Design review of the part built by this model. Coordinates are the model's own, in mm. A direction names the side the tool comes from. Round coordinates to 2 decimals unless told otherwise and drop trailing zeros. Loops run counter-clockwise (first coordinate to the right, second up) from the corner with the lowest first, then second, coordinate; pieces in that order, holes last. Notation, with made-up numbers: M 10,-29.75 L 41,-29.75 A37 ccw 41,9.25 Z; hole C 9,61 d8. An arc over 180 degrees is marked long. One line per item, written item: value. Start each with the question number.
Item 1: We need section A-A (x = 0). Write out the cut boundary in (y, z), then the cut area to 3 significant figures.
Item 2: Clearance check with flat-ended pins moving along their axes: pin 1 (3 mm diameter, centred on y = -6, z = 4.5, fed in from +X); pin 2 (2 mm diameter, centred on y = -6.5, z = 5, fed in from -X); pin 3 (6 mm diameter, centred on x = 8, z = 2.5, fed in from +Y). State where each tip first meets the part, or that it passes through.
Item 3: For faces 1 (the flat face through (3.4, -1.7, 10)), 2 (the cylindrical face through (-2.17, -9.76, 3.94)), list the 3-axis set-ups (+Z, -Z, +X, -X, +Y, -Y) from which the entire face can be reached by the end or side of a thin tool; tool diameter is ignored.
Item 4: For line 1 along Y through (x, z) = (0, 3.75); line 2 along X through (y, z) = (0, -2.1), list the stretches that pass through material, from the lowest coordinate up.
Item 5: Mouldability with a two-part tool opening along Z and no side actions: class faces 3 (the cylindrical face through (-1.08, 4.88, -2.49)), 4 (the flat face through (-0.1, 5.2, -2)), 5 (the flat face through (-5, -9, 0)) as released by +Z, released by -Z, zero draft, split by the parting line, or undercut.
Item 6: We need section D-D (z = -0.5). Write out the cut boundary in (x, y), then the cut area to 3 significant figures.
Item 7: We need section C-C (z = 3.75). Write out the cut boundary in (x, y), then the cut area to 3 significant figures.
from build123d import *

# Parameters (mm, degrees)
F0_R      = 10
F1_DEPTH  = 8
F2_R      = 12
F2_R_2    = 10
F3_DEPTH  = 2
F4_R      = 12
F4_R_2    = 10
F5_DEPTH  = 2
F6_R      = 3
F7_DEPTH  = 25
F9_R      = 5
F9_R_2    = 3
F10_DEPTH = 1
F11_R     = 0.5
F13_R     = 0.5


# Not quite as in the source:
# - a fillet or chamfer that OpenCascade refuses, or shapes differently, is made with other operations: its cross-section is extruded or revolved along the edge and cut away or added


with BuildPart() as f1:
    # F0 (on Top) → F1 (new body)
    with BuildSketch(Plane.XY):
        Circle(F0_R)
    extrude(amount=F1_DEPTH)

    # F2 (on face) → F3 (join)
    with BuildSketch(Plane.XY.offset(8)):
        Circle(F2_R)
        Circle(F2_R_2, mode=Mode.SUBTRACT)
        Circle(F2_R_2)
    extrude(amount=F3_DEPTH)

    # F4 (on face) → F5 (join)
    with BuildSketch(Plane(origin=(0, 0, 0), x_dir=(1, 0, 0), z_dir=(0, 0, -1))):
        Circle(F4_R)
        Circle(F4_R_2, mode=Mode.SUBTRACT)
        Circle(F4_R_2)
    extrude(amount=F5_DEPTH)

    # F6 (on face) → F7 (cut)
    with BuildSketch(Plane(origin=(0, 0, -2), x_dir=(1, 0, 0), z_dir=(0, 0, -1))):
        Circle(F6_R)
    extrude(amount=-F7_DEPTH, mode=Mode.SUBTRACT)

    # F8: union 

    # F9 (on face) → F10 (join)
    with BuildSketch(Plane(origin=(0, 0, -2), x_dir=(1, 0, 0), z_dir=(0, 0, -1))):
        Circle(F9_R)
        Circle(F9_R_2, mode=Mode.SUBTRACT)
    extrude(amount=F10_DEPTH)

    # F11
    f11_edges = [f1.edges().sort_by_distance(p)[0] for p in [
        (-3, 0, -3),
    ]]
    fillet(f11_edges, radius=F11_R)

    # F12: fillet of radius 5 on 2 edges, made by hand

    # F12_s1 → F12_t2 (revolve, cut)
    with BuildSketch(Plane.XZ):
        with BuildLine():
            ThreePointArc((8, -2), (10.2360679775, -1.472135955), (12, 0))
            Line((12, 0), (12, -2))
            Line((12, -2), (8, -2))
        make_face()
    revolve(axis=Axis((0, 0, -2), (0, 0, -1)), mode=Mode.SUBTRACT)

    # F12_s3 → F12_t4 (revolve, cut)
    with BuildSketch(Plane.XZ):
        with BuildLine():
            ThreePointArc((8, 10), (10.2360679775, 9.472135955), (12, 8))
            Line((12, 8), (12, 10))
            Line((12, 10), (8, 10))
        make_face()
    revolve(axis=Axis((0, 0, 10), (0, 0, 1)), mode=Mode.SUBTRACT)

    # F13
    f13_edges = [f1.edges().sort_by_distance(p)[0] for p in [
        (3, 0, 4),
        (-3, 0, 10),
        (-3, 0, -2),
        (3, 0, -2.25),
        (-3, 0, -2.5),
    ]]
    fillet(f13_edges, radius=F13_R)


solid = f1.part
A:
1. outline: M -12,0 A5 ccw -8,-2 L -5,-2 L -5,-3 L -3.5,-3 A0.5 ccw -3,-2.5 L -3,9.5 A0.5 ccw -3.5,10 L -8,10 A5 ccw -12,8 L -10,8 L -10,0 Z; M 3,-2.5 A0.5 ccw 3.5,-3 L 5,-3 L 5,-2 L 8,-2 A5 ccw 12,0 L 10,0 L 10,8 L 12,8 A5 ccw 8,10 L 3.5,10 A0.5 ccw 3,9.5 Z
1. area: 178 mm2
2. pin 1: x = 8.93
2. pin 2: x = -8.35
2. pin 3: y = 10.19
3. face 1: +Z, +X, -X, +Y, -Y
3. face 2: none
4. line 1: -10 to -3, 3 to 10
4. line 2: -5 to -3, 3 to 5
5. face 3: zero draft
5. face 4: released by -Z
5. face 5: undercut
6. outline: C 0,0 d23.14; hole C 0,0 d6
6. area: 392 mm2
7. outline: C 0,0 d20; hole C 0,0 d6
7. area: 286 mm2
